```python
from build123d import *


with BuildPart() as f1:
    # F0 (on Front) → F1 (revolve)
    with BuildSketch(Plane.XZ):
        with BuildLine():
            ThreePointArc((2, -4), (2.236068, -1.381966), (0, 0))
            Line((0, 0), (0, -75))
            Line((0, -75), (15, -75))
            Line((15, -75), (15, -72))
            Line((15, -72), (12.002306, -70))
            ThreePointArc((12.002306, -70), (12.689754, -64.782464), (9, -61.03))
            Line((9, -61.03), (9, -60.03))
            ThreePointArc((9, -60.03), (8.732051, -59.03), (8, -58.297949))
            Line((8, -58.297949), (7.5, -58.297949))
            ThreePointArc((7.5, -58.297949), (4.666942, -42.583339), (7.5, -26.868728))
            Line((7.5, -26.868728), (8.83642, -26.868728))
            ThreePointArc((8.83642, -26.868728), (9.940865, -24.645891), (8.031478, -23.06))
            ThreePointArc((8.031478, -23.06), (7.56805, -12.722329), (2, -4))
        make_face()
    revolve(axis=Axis((0, 0, -37.5), (0, 0, -1)))


solid = f1.part
```
Check sheet for the modelled part. Datum: model origin and axes. Units: mm. Round coordinates to 2 decimals unless told otherwise and drop trailing zeros. Order: outer loops, then holes, each group sorted by start corner. A loop starts at its lowest first (then second) coordinate and runs counter-clockwise, first axis right, second up.
1) Scan lines: line 1 (Z direction, x = -2.25, y = -0.5); line 2 (Z direction, x = 5.5, y = 7.75); line 3 (X direction, y = -1.25, z = -31). Record each from-to range of solid material in increasing order.
2) Section check A-A (z = -41.5). Record the boundary of the cut face in (x, y), and give its area (3 significant figures).
3) Go/stop test with flat-tipped pins: pin 1 Ø3 at (x, z) = (5.5, -33) entering from +Y; pin 2 Ø5 at (x, z) = (-4, -35) entering from -Y; pin 3 Ø6 at (x, z) = (-4.5, -51) entering from -Y. Record where each tip stops, or that it passes through.
4) Mould release check, pull along Z, two halves, no side actions. Record for faces 1 (the flat face through (0, 0, -75)), 2 (the cylindrical face through (-14.985, -0.66, -73.479)), 3 (the flat face through (4, 7, -26.869)): +Z half, -Z half, draft (parallel to the pull), parting line (faces both ways), or undercut.
5) Section check B-B (z = -50.5). Record the boundary of the cut face in (x, y).
Result:
1. line 1: z = -75 to -4.28, -3.47 to -1.53
1. line 2: z = -75 to -61.23, -26.36 to -23.76
1. line 3: x = -6.06 to 6.06
2. outline: circle Ø9.36 at (0, 0)
2. area: 68.8 mm2
3. pin 1: stops at y = 4.13
3. pin 2: stops at y = -5.23
3. pin 3: stops at y = -5.45
4. face 1: -Z half
4. face 2: draft
4. face 3: undercut
5. outline: circle Ø10.74 at (0, 0)
